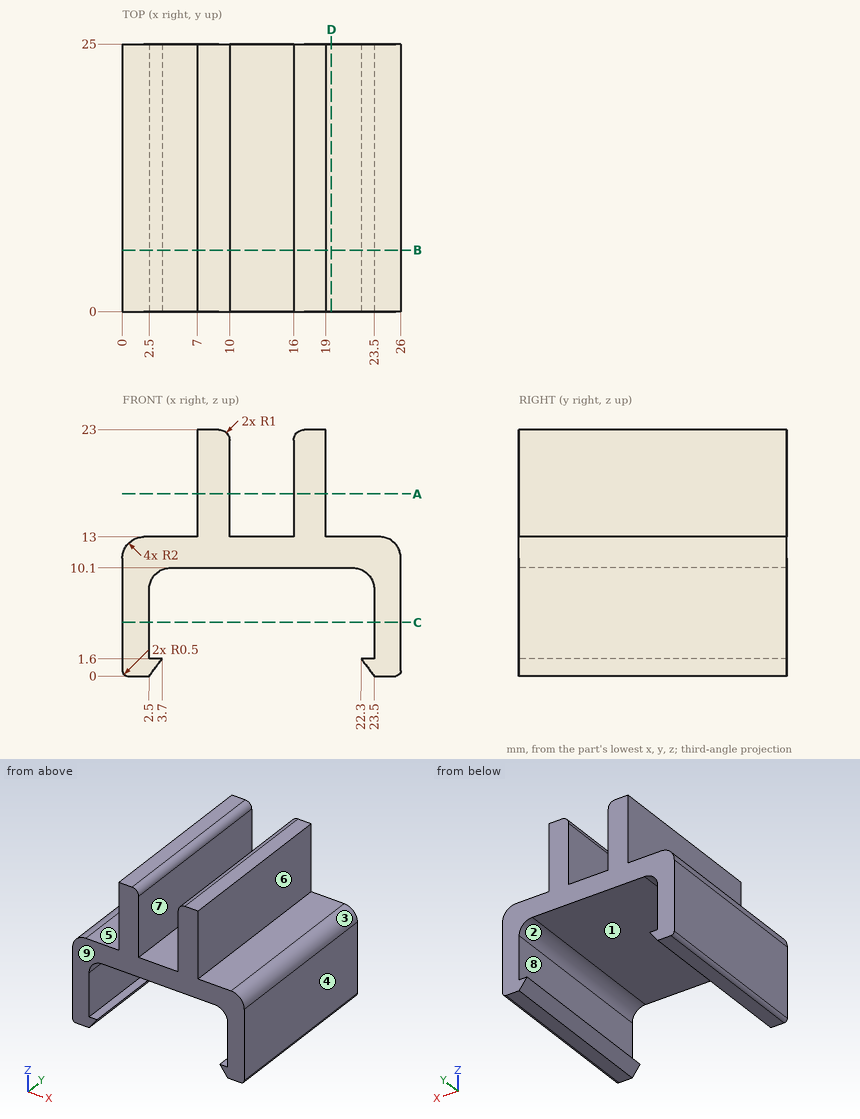
Job drawing, mm, ordinate dimensions from the low corner. One solid piece. A direction names the side the tool comes from. Round coordinates to 2 decimals unless told otherwise and drop trailing zeros. Write each loop counter-clockwise with the first axis right and the second up, starting at its lowest first coordinate (ties: lowest second). Pieces come first, ordered by that corner, then holes. Notation, with made-up numbers: (-1, 87.5) -> (57, 87.5) arc R14 cw to (57, 92.5) -> close; hole circle Ø7 at (71.5, 25.5). An arc over 180 degrees is marked (long way). Answer as a JSON object with one key per item and string values.
(1) Band-saw the part on B-B, the plane y = 5.75. List the corners of the cut face in (x, z).
Reported:
{"outline": "(0, 0.5) arc R0.5 ccw to (0.5, 0) -> (2.5, 0) -> (3.7, 1.6) -> (2.5, 1.6) -> (2.5, 8.1) arc R2 cw to (4.5, 10.1) -> (21.5, 10.1) arc R2 cw to (23.5, 8.1) -> (23.5, 1.6) -> (22.3, 1.6) -> (23.5, 0) -> (25.5, 0) arc R0.5 ccw to (26, 0.5) -> (26, 11) arc R2 ccw to (24, 13) -> (19, 13) -> (19, 23) -> (17, 23) arc R1 ccw to (16, 22) -> (16, 13) -> (10, 13) -> (10, 22) arc R1 ccw to (9, 23) -> (7, 23) -> (7, 13) -> (2, 13) arc R2 ccw to (0, 11) -> close"}
(2) Pin check, flat tips, straight feed: P1, Ø13.5, axis at x = 11.5, y = 17, coming from the -Z side; P2, Ø4.5, axis at y = 15, z = 18.5, coming from the -X side; P3, Ø4.5, axis at y = 10.5, z = 17.5, coming from the +X side. Stop position of each tip, or through.
Reported:
{"P1": "stops at z = 10.1", "P2": "stops at x = 7", "P3": "stops at x = 19"}
(3) Band-saw the part on C-C, the plane z = 5. List the corners of the cut face in (x, y).
Reported:
{"outline": "(0, 0) -> (2.5, 0) -> (2.5, 25) -> (0, 25) -> close; (23.5, 0) -> (26, 0) -> (26, 25) -> (23.5, 25) -> close"}
(4) Band-saw the part on D-D, the plane x = 19.5. List the corners of the cut face in (y, z), then the cut area to 3 significant figures.
Reported:
{"outline": "(0, 10.1) -> (25, 10.1) -> (25, 13) -> (0, 13) -> close", "area": "72.5 mm^2"}
(5) Band-saw the part on A-A, the plane z = 17. List the corners of the cut face in (x, y), then the cut area to 3 significant figures.
Reported:
{"outline": "(7, 0) -> (10, 0) -> (10, 25) -> (7, 25) -> close; (16, 0) -> (19, 0) -> (19, 25) -> (16, 25) -> close", "area": "150 mm^2"}
(6) Which spindle directions (+Z, -Z, +X, -X, +Y, -Y) get a long thin tool onto all of the face, cutting with end or side? Do the marked faces 5, 6, 7, 8 and 9. Say none if no direction does.
Reported:
{"face 5": "+Z, -X, +Y, -Y", "face 6": "+Z, +X, +Y, -Y", "face 7": "+Z, +Y, -Y", "face 8": "+Y, -Y", "face 9": "+Z, -Z, +X, -X, -Y"}
(7) Probe probe 1 along X at (y, z) = (17.25, 3); probe 2 along X at (y, z) = (14.25, 20.75); probe 3 along Z at (x, y) = (17.5, 21.25). List the from-to ranges inside material, lowest first. Write a range as [from, to].
Reported:
{"probe 1": "x = [0, 2.5], [23.5, 26]", "probe 2": "x = [7, 10], [16, 19]", "probe 3": "z = [10.1, 23]"}
(8) Two-plate mould, pull along Z, no slides. Class the marked faces 1, 2, 3 and 4: +Z half, -Z half, draft (parallel to the pull), parting line (faces both ways), or undercut.
Reported:
{"face 1": "-Z half", "face 2": "undercut", "face 3": "+Z half", "face 4": "draft"}
